Drawing for the job (mm, zero at the part's lowest x, y, z). Give positions to 0.01 mm unless a question says otherwise; leave off trailing zeros. Order: outer loops, then holes, each group sorted by start corner. A loop starts at its lowest first (then second) coordinate and runs counter-clockwise, first axis right, second up. Notation, with made-up numbers: (25.5, 64) - (83.5, 64) arc R24 cw to (83.5, 96) - close; hole circle Ø9 at (8.5, 82). An arc over 180 degrees is marked (long way). Use a Markdown table: item, result.
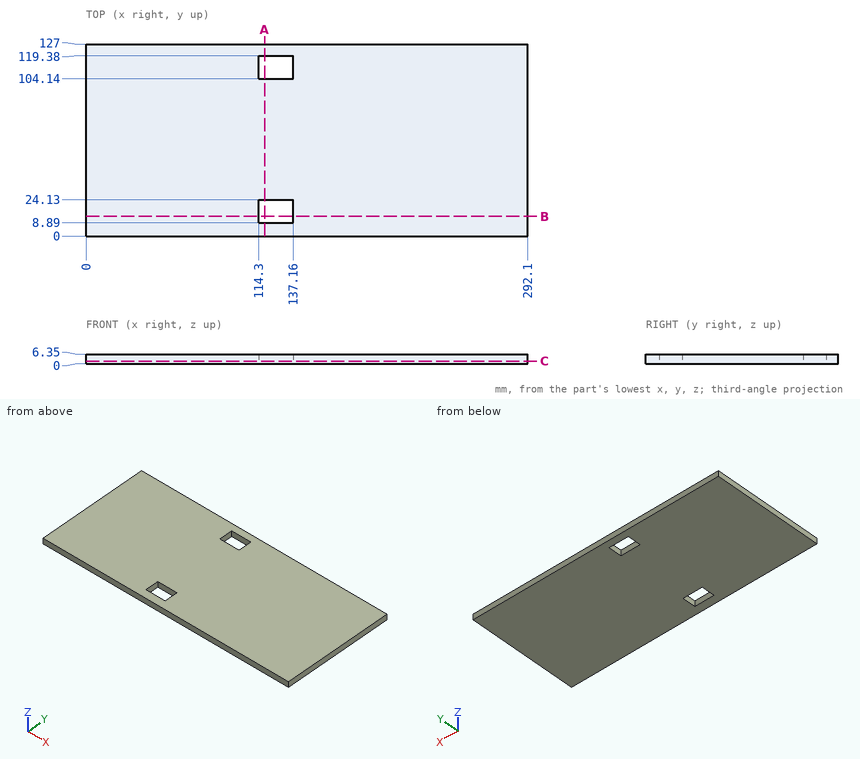
1) Slice it at B-B (y = 13). Write the cut outline in (x, z), and give its area (3 significant figures).
Computed:
| item | result |
|---|---|
| outline | (0, 0) - (114.3, 0) - (114.3, 6.35) - (0, 6.35) - close; (137.16, 0) - (292.1, 0) - (292.1, 6.35) - (137.16, 6.35) - close |
| area | 1,710 mm² |
2) Slice it at A-A (x = 118). Write the cut outline in (y, z).
Computed:
| item | result |
|---|---|
| outline | (0, 0) - (8.89, 0) - (8.89, 6.35) - (0, 6.35) - close; (24.13, 0) - (104.14, 0) - (104.14, 6.35) - (24.13, 6.35) - close; (119.38, 0) - (127, 0) - (127, 6.35) - (119.38, 6.35) - close |
3) Slice it at C-C (z = 1.75). Write the cut outline in (x, y).
Computed:
| item | result |
|---|---|
| outline | (0, 0) - (292.1, 0) - (292.1, 127) - (0, 127) - close; hole (114.3, 8.89) - (137.16, 8.89) - (137.16, 24.13) - (114.3, 24.13) - close; hole (114.3, 104.14) - (137.16, 104.14) - (137.16, 119.38) - (114.3, 119.38) - close |
4) Wall check: line 1 (X direction, y = 22.5, z = 4.75); line 2 (Y direction, x = 128, z = 6.25). Give the ranges that are in metal, low to high. Write a range as from..to.
Computed:
| item | result |
|---|---|
| line 1 | x = 0..114.3, 137.16..292.1 |
| line 2 | y = 0..8.89, 24.13..104.14, 119.38..127 |
